Source: three-view drawing plus pictorial views. Frame: mm from the lowest corner of the part. Give positions to 0.01 mm unless a question says otherwise; leave off trailing zeros. Write each loop counter-clockwise with the first axis right and the second up, starting at its lowest first coordinate (ties: lowest second). Pieces come first, ordered by that corner, then holes. Notation, with made-up numbers: (44, 24) -> (89, 24) arc R23 cw to (89, 58) -> close; hole circle Ø11 at (33.25, 56). An arc over 180 degrees is marked (long way). Write item = value, one per line.
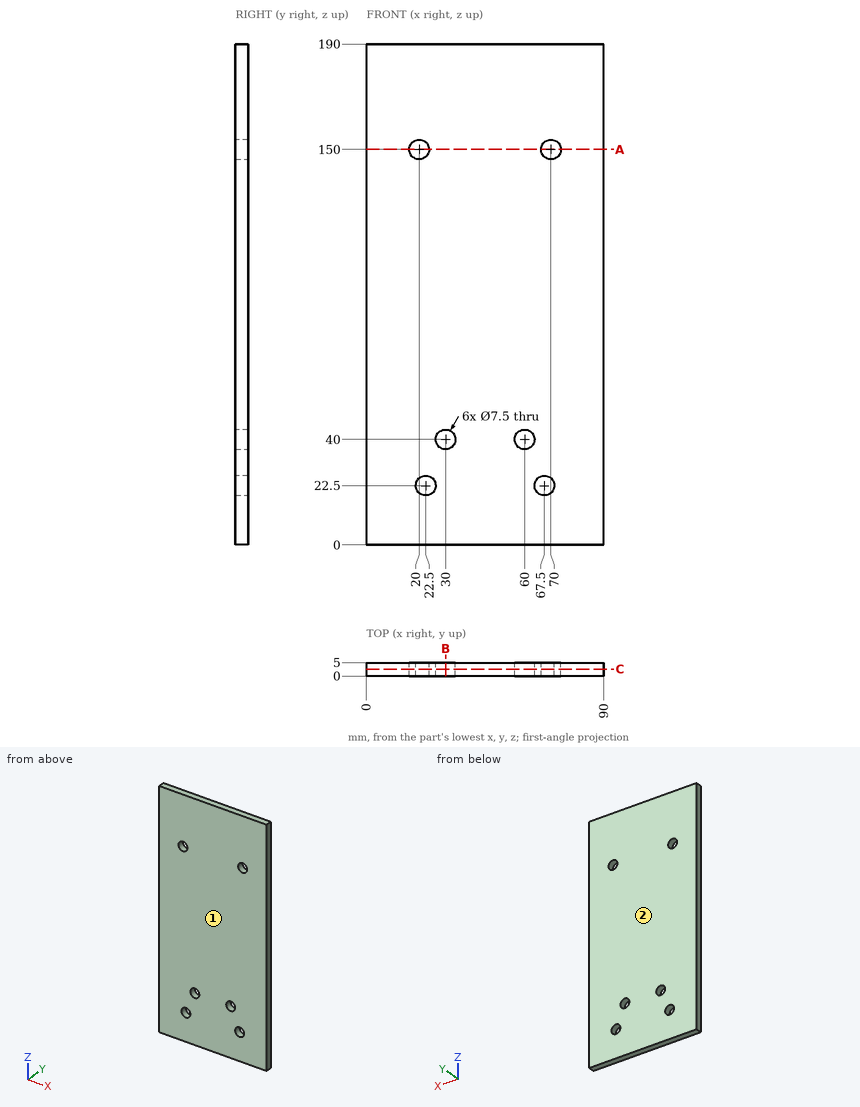
1) Cut plane B-B (x = 30). Return the cut outline in (y, z), then the cut area to 4 significant figures.
Computed:
outline = (0, 0) -> (5, 0) -> (5, 36.25) -> (0, 36.25) -> close; (0, 43.75) -> (5, 43.75) -> (5, 190) -> (0, 190) -> close
area = 912.5 mm²
2) Draft query along Y for the marked faces 1 and 2. Return one class per face: pulls with the +Y half, pulls with the -Y half, needs draft (parallel to the pull), parting line crosses it, or undercut.
Computed:
face_1 = pulls with the -Y half
face_2 = pulls with the +Y half
3) Cut plane A-A (z = 150). Return the cut outline in (x, y), then the cut area to 3 significant figures.
Computed:
outline = (0, 0) -> (16.25, 0) -> (16.25, 5) -> (0, 5) -> close; (23.75, 0) -> (66.25, 0) -> (66.25, 5) -> (23.75, 5) -> close; (73.75, 0) -> (90, 0) -> (90, 5) -> (73.75, 5) -> close
area = 375 mm²
4) Cut plane C-C (y = 2.6). Return the cut outline in (x, z), then the cut area to 3 significant figures.
Computed:
outline = (0, 0) -> (90, 0) -> (90, 190) -> (0, 190) -> close; hole circle Ø7.5 at (20, 150); hole circle Ø7.5 at (22.5, 22.5); hole circle Ø7.5 at (30, 40); hole circle Ø7.5 at (60, 40); hole circle Ø7.5 at (67.5, 22.5); hole circle Ø7.5 at (70, 150)
area = 16,800 mm²
5) Contact query for flat-ended pins moving along their axis: pin 1 (7 mm diameter, centred on x = 60, z = 40, fed in from +Y); pin 2 (10 mm diameter, centred on x = 30, z = 40, fed in from -Y). Output: stop coordinate, or through.
Computed:
pin_1 = through
pin_2 = 0
6) Material intervals for L1, parallel to X at y = 1.75, z = 23; L2, parallel to X at y = 3.55, z = 150; L3, parallel to Z at x = 18.5, y = 2.35, sorted ascending.
Computed:
L1 = 0 to 18.78, 26.22 to 63.78, 71.22 to 90
L2 = 0 to 16.25, 23.75 to 66.25, 73.75 to 90
L3 = 0 to 146.56, 153.44 to 190
